Here's the drawing with two shaded views (mm, measured from the low corner). I have some questions. A direction names the side the tool comes from. Give positions to 0.01 mm unless a question says otherwise; leave off trailing zeros. Order: outer loops, then holes, each group sorted by start corner. A loop starts at its lowest first (then second) coordinate and runs counter-clockwise, first axis right, second up. Notation, with made-up numbers: M 89,-33 L 118,-33 A38 cw 118,6 Z; hole C -19.5,32.25 d10. An arc over 180 degrees is marked long. Use a Markdown table: item, result. Add a question column.
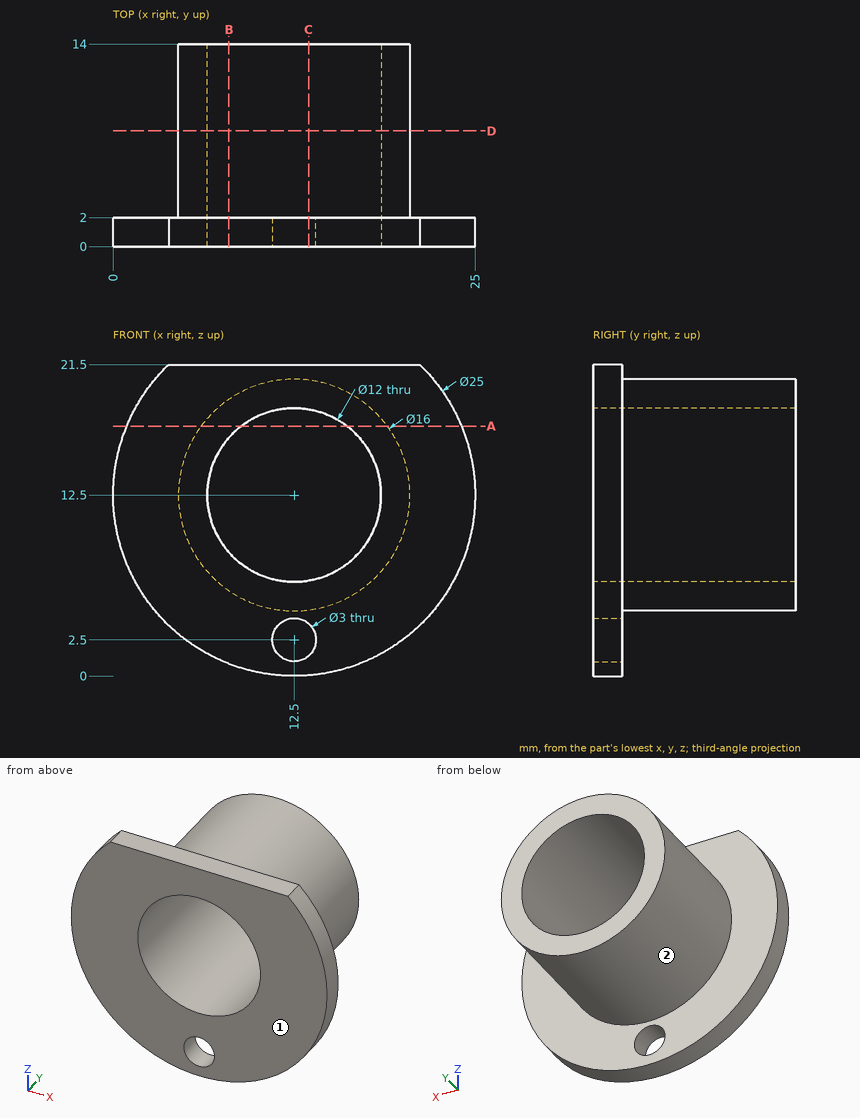
1. I need wall thicknesses on L1, parallel to Z at x = 11.25, y = 1; L2, parallel to Z at x = 12.25, y = 9.5; L3, parallel to Y at x = 18.5, z = 5.25. Which ranges of each line are inside material? Lowest first, please. Write a range as [from, to].
2. Will these pins go through, and if not, where does the flat tip stop? pin 1 (8 mm diameter, centred on x = 17, z = 5, fed in from +Y); pin 2 (1.5 mm diameter, centred on x = 16.5, y = 10.5, fed in from +Z); pin 3 (1 mm diameter, centred on x = 9.5, y = 9, fed in from -Z); pin 4 (8 mm diameter, centred on x = 15.5, y = 8, fed in from +Z).
3. If we section it at D-D, the plane y = 8: List the corners of the cut face in (x, z) for me, then the cut area to 3 significant figures.
4. On a 3-axis mill with a long thin cutter (end or side, diameter ignored), from which of +Z, -Z, +X, -X, +Y, -Y can I reach the whole of each face in a straight line? I mean the marked faces 1 and 2. Say none if no direction works.
5. If we section it at A-A, the plane z = 17.25: List the corners of the cut face in (x, y) for me, then the cut area to 3 significant figures.
6. If we section it at B-B, the plane x = 8: List the corners of the cut face in (y, z) for me.
7. If we section it at C-C, the plane x = 13.5: List the corners of the cut face in (y, z) for me.
Geometry results:
| question | item | result |
|---|---|---|
| 1 | L1 | z = [0.06, 1.67], [3.33, 6.63], [18.37, 21.5] |
| 1 | L2 | z = [4.5, 6.51], [18.49, 20.5] |
| 1 | L3 | y = [0, 2] |
| 2 | pin 1 | stops at y = 14 |
| 2 | pin 2 | stops at z = 19.81 |
| 2 | pin 3 | stops at z = 4.9 |
| 2 | pin 4 | stops at z = 20.5 |
| 3 | outline | C 12.5,12.5 d16; hole C 12.5,12.5 d12 |
| 3 | area | 88.0 mm^2 |
| 4 | face 1 | +Z, -Z, +X, -X, -Y |
| 4 | face 2 | +Y |
| 5 | outline | M 0.94,0 L 8.83,0 L 8.83,14 L 6.06,14 L 6.06,2 L 0.94,2 Z; M 16.17,0 L 24.06,0 L 24.06,2 L 18.94,2 L 18.94,14 L 16.17,14 Z |
| 5 | area | 98.1 mm^2 |
| 6 | outline | M 0,0.84 L 2,0.84 L 2,5.89 L 14,5.89 L 14,8.53 L 0,8.53 Z; M 0,16.47 L 14,16.47 L 14,19.11 L 2,19.11 L 2,21.5 L 0,21.5 Z |
| 7 | outline | M 0,0.04 L 2,0.04 L 2,1.38 L 0,1.38 Z; M 0,3.62 L 2,3.62 L 2,4.56 L 14,4.56 L 14,6.58 L 0,6.58 Z; M 0,18.42 L 14,18.42 L 14,20.44 L 2,20.44 L 2,21.5 L 0,21.5 Z |
